Geometry: final body of the model. Coordinates: model frame, mm. A direction names the side the tool comes from. Round coordinates to 2 decimals unless told otherwise and drop trailing zeros. Loops run counter-clockwise (first coordinate to the right, second up) from the corner with the lowest first, then second, coordinate; pieces in that order, holes last. Notation, with made-up numbers: M 13,-28 L 54,-28 A9 ccw 54,-18 Z; hole C 52,75.5 d11. An arc over 180 degrees is marked long. Write each question's results on one line, items separated by ' | '.
```python
from build123d import *

# Parameters (mm, degrees)
ESQUISSE1_R             = 1
EXTRUSION1_DEPTH        = 5
ESQUISSE2_R             = 1.259960856
ENL_V_MAT_EXTRU_1_DEPTH = 15
ESQUISSE3_R             = 2
ENL_V_MAT_EXTRU_2_DEPTH = 3


with BuildPart() as part:
    # Esquisse1 → Extrusion1 (new body)
    with BuildSketch(Plane.XY):
        with BuildLine():
            Line((-30.206178794, 71.120250568), (-30.206178794, 59.916517686))
            ThreePointArc((-30.206178794, 59.916517686), (-27.371580774, 57.081919667), (-24.536982754, 59.916517686))
            Line((-24.536982754, 59.916517686), (-24.536982754, 71.120250568))
            ThreePointArc((-24.536982754, 71.120250568), (-27.371580774, 73.954848588), (-30.206178794, 71.120250568))
        make_face()
        with Locations((-27.371580774, 59.916517686)):
            Circle(ESQUISSE1_R, mode=Mode.SUBTRACT)
        with Locations((-27.371580774, 71.120250568)):
            Circle(ESQUISSE1_R, mode=Mode.SUBTRACT)
        with BuildLine():
            Line((-29.038880927, 68.862401416), (-29.038880927, 62.190489948))
            ThreePointArc((-29.038880927, 62.190489948), (-27.330220673, 63.062743756), (-25.621560419, 62.190489948))
            Line((-25.621560419, 62.190489948), (-25.621560419, 68.862401416))
            ThreePointArc((-25.621560419, 68.862401416), (-27.330220673, 67.980247638), (-29.038880927, 68.862401416))
        make_face(mode=Mode.SUBTRACT)
    extrude(amount=EXTRUSION1_DEPTH)

    # Esquisse2 → Enlèv. mat.-Extru.1 (cut)
    with BuildSketch(Plane(origin=(-24.536982754, 0, 0), x_dir=(0, 0, -1), z_dir=(1, 0, 0))):
        with Locations((0, 65.518384127)):
            Circle(ESQUISSE2_R)
    extrude(amount=-ENL_V_MAT_EXTRU_1_DEPTH, mode=Mode.SUBTRACT)

    # Esquisse3 → Enlèv. mat.-Extru.2 (cut)
    with BuildSketch(Plane(origin=(0, 0, 0), x_dir=(-1, 0, 0), z_dir=(0, 0, -1))):
        with Locations((27.371580774, 71.120250568)):
            Circle(ESQUISSE3_R)
        with Locations((27.371580774, 59.916517686)):
            Circle(ESQUISSE3_R)
    extrude(amount=-ENL_V_MAT_EXTRU_2_DEPTH, mode=Mode.SUBTRACT)


solid = part.part
```
1. Section D-D (x = -27.85). Output: boundary loops of the cut face in (y, z), then the cut area to 3 significant figures.
Answer key:
outline: M 57.12,0 L 57.97,0 L 57.97,3 L 59.04,3 L 59.04,5 L 57.12,5 Z; M 60.79,3 L 61.86,3 L 61.86,0 L 63,0 L 63,5 L 60.79,5 Z; M 68.05,0 L 69.18,0 L 69.18,3 L 70.24,3 L 70.24,5 L 68.05,5 Z; M 72,3 L 73.06,3 L 73.06,0 L 73.91,0 L 73.91,5 L 72,5 Z | area: 28.4 mm²
2. Section B-B (z = 4.45). Output: boundary loops of the cut face in (x, y).
Answer key:
outline: M -30.21,59.92 A2.83 ccw -24.54,59.92 L -24.54,71.12 A2.83 ccw -30.21,71.12 Z; hole M -29.04,62.19 A2.11 cw -25.62,62.19 L -25.62,68.86 A2.1 cw -29.04,68.86 Z; hole C -27.37,59.92 d2; hole C -27.37,71.12 d2
3. Draft query along Y for faces 1 (the face through (-30.206, 66, 2)), 2 (the face through (-27.309, 73.954, 2.465)), 3 (the face through (-27.5, 72.11, 3.99)). Return one class per face: pulls with the +Y half, pulls with the -Y half, needs draft (parallel to the pull), parting line crosses it, or undercut.
Answer key:
face 1: needs draft | face 2: pulls with the +Y half | face 3: undercut
4. Pin query (flat end, axial travel): P1, Ø2.5, axis at x = -27.37, y = 71.12, coming from the -Z side; P2, Ø3, axis at x = -26, z = 1.5, coming from the +Y side. Return the tip coordinate at first contact, or that it passes through.
Answer key:
P1: stops at z = 3 | P2: stops at y = 73.95
5. Ray query, probe 1 along X at (y, z) = (63.5, 3.95); probe 2 along X at (y, z) = (71, 2.65); probe 3 along X at (y, z) = (68.25, 1.8). Return the intervals inside material, ascending.
Answer key:
probe 1: x = -30.21 to -29.04, -25.62 to -24.54 | probe 2: x = -30.21 to -29.37, -25.38 to -24.54 | probe 3: x = -30.21 to -29.04, -28.36 to -26.3, -25.62 to -24.54
6. Section C-C (x = -28.85). Output: boundary loops of the cut face in (y, z).
Answer key:
outline: M 57.5,0 L 58.57,0 L 58.57,3 L 61.26,3 L 61.26,0 L 62.42,0 L 62.42,5 L 57.5,5 Z; M 68.63,0 L 69.77,0 L 69.77,3 L 72.47,3 L 72.47,0 L 73.54,0 L 73.54,5 L 68.63,5 Z
7. Access query for faces 4 (the face through (-25.622, 65, 2)), 5 (the face through (-26, 62, 0)), 6 (the face through (-26, 71, 3)). Directions: +Z, -Z, +X, -X, +Y, -Y. A direction counts if a zero-diameter tool reaches every point of the face in a straight line with its end or side. Return the directions, or none.
Answer key:
face 4: +Z, -Z | face 5: -Z, +X, -X, +Y, -Y | face 6: -Z
8. Section A-A (y = 64). Output: boundary loops of the cut face in (x, z).
Answer key:
outline: M -30.21,0 L -29.04,0 L -29.04,5 L -30.21,5 Z; M -25.62,0 L -24.54,0 L -24.54,5 L -25.62,5 Z
